The listing builds one solid part. Answer for the finished solid, in the listing's coordinates (mm). Face numbers are marked on the shaded views. A direction names the side the tool comes from. Coordinates: 2 decimals unless noted, no trailing zeros. Write each loop counter-clockwise with the first axis right and the second up, starting at its lowest first coordinate (ties: lowest second). Pieces come first, ordered by that corner, then holes.
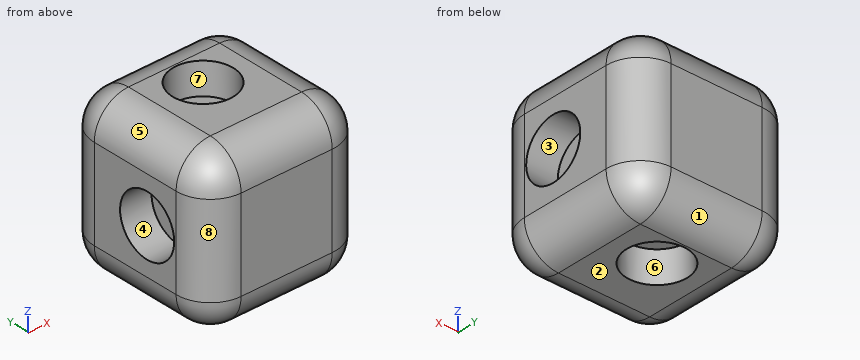
from build123d import *

# Parameters (mm, degrees)
SKETCH1_W                = 29.6037
SKETCH1_H                = 29.6037
BOSS_EXTRUDE1_DEPTH      = 14.80185
BOSS_EXTRUDE1_DEPTH_BACK = 14.80185
FILLET3_R                = 6.35
FILLET4_R                = 6.35
FILLET5_R                = 6.35
FILLET6_R                = 6.35
SKETCH7_R                = 5.588
CUT_EXTRUDE3_DEPTH       = 5.842
SKETCH8_R                = 5.588
CUT_EXTRUDE4_DEPTH       = 5.842
SKETCH3_R                = 5.588
CUT_EXTRUDE5_DEPTH       = 5.842
SKETCH9_R                = 5.588
CUT_EXTRUDE6_DEPTH       = 5.842
FILLET7_R                = 6.35
FILLET8_R                = 6.35


with BuildPart() as part:
    # Sketch1 → Boss-Extrude1 (new body, two sides)
    with BuildSketch(Plane.XY) as boss_extrude1_sk:
        Rectangle(SKETCH1_W, SKETCH1_H)
    extrude(amount=BOSS_EXTRUDE1_DEPTH)
    extrude(boss_extrude1_sk.sketch, amount=-BOSS_EXTRUDE1_DEPTH_BACK)

    # Fillet3
    fillet3_edges = [part.edges().sort_by_distance(p)[0] for p in [
        (14.80185, 14.80185, 0),
    ]]
    fillet(fillet3_edges, radius=FILLET3_R)

    # Fillet4
    fillet4_edges = [part.edges().sort_by_distance(p)[0] for p in [
        (-14.80185, 14.80185, 0),
    ]]
    fillet(fillet4_edges, radius=FILLET4_R)

    # Fillet5
    fillet5_edges = [part.edges().sort_by_distance(p)[0] for p in [
        (-14.80185, -14.80185, 0),
    ]]
    fillet(fillet5_edges, radius=FILLET5_R)

    # Fillet6
    fillet6_edges = [part.edges().sort_by_distance(p)[0] for p in [
        (14.80185, -14.80185, 0),
    ]]
    fillet(fillet6_edges, radius=FILLET6_R)

    # Sketch7 → Cut-Extrude3 (cut)
    with BuildSketch(Plane(origin=(0, 0, -14.80185), x_dir=(-1, 0, 0), z_dir=(0, 0, -1))):
        with Locations((0, 2.47015)):
            Circle(SKETCH7_R)
    extrude(amount=-CUT_EXTRUDE3_DEPTH, mode=Mode.SUBTRACT)

    # Sketch8 → Cut-Extrude4 (cut)
    with BuildSketch(Plane.XY.offset(14.80185)):
        with Locations((0, 2.47015)):
            Circle(SKETCH8_R)
    extrude(amount=-CUT_EXTRUDE4_DEPTH, mode=Mode.SUBTRACT)

    # Sketch3 → Cut-Extrude5 (cut)
    with BuildSketch(Plane.ZY.offset(14.80185)):
        with Locations((0, -2.47015)):
            Circle(SKETCH3_R)
    extrude(amount=-CUT_EXTRUDE5_DEPTH, mode=Mode.SUBTRACT)

    # Sketch9 → Cut-Extrude6 (cut)
    with BuildSketch(Plane(origin=(14.80185, 0, 0), x_dir=(0, 0, -1), z_dir=(1, 0, 0))):
        with Locations((0, -2.47015)):
            Circle(SKETCH9_R)
    extrude(amount=-CUT_EXTRUDE6_DEPTH, mode=Mode.SUBTRACT)

    # Fillet7
    fillet7_edges = [part.edges().sort_by_distance(p)[0] for p in [
        (0, 14.80185, 14.80185),
        (-14.80185, 0, 14.80185),
        (0, -14.80185, 14.80185),
        (14.80185, 0, 14.80185),
    ]]
    fillet(fillet7_edges, radius=FILLET7_R)

    # Fillet8
    fillet8_edges = [part.edges().sort_by_distance(p)[0] for p in [
        (0, 14.80185, -14.80185),
        (-14.80185, 0, -14.80185),
        (0, -14.80185, -14.80185),
        (14.80185, 0, -14.80185),
    ]]
    fillet(fillet8_edges, radius=FILLET8_R)


solid = part.part
Q1. Which of the six approach directions +Z, -Z, +X, -X, +Y, -Y give full straight-line access (tool end or side, diameter ignored) to the marked faces 4, 5, 6, 7 and 8?
Answers below:
face 4: -X
face 5: +Z, -X, +Y, -Y
face 6: -Z
face 7: +Z
face 8: +Z, -Z, -X, -Y
Q2. The part is cut by section D-D, the plane z = 8. Write down the section's boundary in (x, y), then the cut area to 3 significant figures.
Answers below:
outline: (-14.8, -8.45) arc R6.35 ccw to (-8.45, -14.8) - (8.45, -14.8) arc R6.35 ccw to (14.8, -8.45) - (14.8, 8.45) arc R6.35 ccw to (8.45, 14.8) - (-8.45, 14.8) arc R6.35 ccw to (-14.8, 8.45) - close
area: 842 mm2
Q3. Given pin 1 (10 mm diameter, centred on x = 0, y = 2.47, fed in from -Z); pin 2 (1.5 mm diameter, centred on x = 0.5, y = -9.5, fed in from -Z); pin 3 (3 mm diameter, centred on x = -11.5, z = -2, fed in from +Y), each flat-ended and moving along its own axis, determine where each tip first touches the part or whether it passes through.
Answers below:
pin 1: stops at z = -8.96
pin 2: stops at z = -14.79
pin 3: stops at y = 14.61
Q4. The part is cut by section B-B, the plane x = 0. Write down the section's boundary in (y, z).
Answers below:
outline: (-14.8, -8.45) arc R6.35 ccw to (-8.45, -14.8) - (-3.12, -14.8) - (-3.12, -8.96) - (8.06, -8.96) - (8.06, -14.8) - (8.45, -14.8) arc R6.35 ccw to (14.8, -8.45) - (14.8, 8.45) arc R6.35 ccw to (8.45, 14.8) - (8.06, 14.8) - (8.06, 8.96) - (-3.12, 8.96) - (-3.12, 14.8) - (-8.45, 14.8) arc R6.35 ccw to (-14.8, 8.45) - close
Q5. Find the intervals of material crossed by probe 1 along Y at (x, z) = (0, 11.75); probe 2 along Y at (x, z) = (-1.5, -9); probe 3 along X at (y, z) = (1.5, -12), in increasing order.
Answers below:
probe 1: y = -13.88 to -3.12, 8.06 to 13.88
probe 2: y = -14.78 to -2.91, 7.85 to 14.78
probe 3: x = -13.72 to -5.5, 5.5 to 13.72
Q6. Determine the mould class of the marked faces 1, 2 and 3 for opening direction Y: released by +Y, released by -Y, zero draft, split by the parting line, or undercut.
Answers below:
face 1: released by +Y
face 2: zero draft
face 3: undercut
Q7. The part is cut by section A-A, the plane z = 0. Write down the section's boundary in (x, y), then the cut area to 3 significant figures.
Answers below:
outline: (-14.8, -8.45) arc R6.35 ccw to (-8.45, -14.8) - (8.45, -14.8) arc R6.35 ccw to (14.8, -8.45) - (14.8, -8.06) - (8.96, -8.06) - (8.96, 3.12) - (14.8, 3.12) - (14.8, 8.45) arc R6.35 ccw to (8.45, 14.8) - (-8.45, 14.8) arc R6.35 ccw to (-14.8, 8.45) - (-14.8, 3.12) - (-8.96, 3.12) - (-8.96, -8.06) - (-14.8, -8.06) - close
area: 711 mm2
Q8. The part is cut by section C-C, the plane y = 0. Write down the section's boundary in (x, z), then the cut area to 3 significant figures.
Answers below:
outline: (-14.8, -8.45) arc R6.35 ccw to (-8.45, -14.8) - (-5.01, -14.8) - (-5.01, -8.96) - (5.01, -8.96) - (5.01, -14.8) - (8.45, -14.8) arc R6.35 ccw to (14.8, -8.45) - (14.8, -5.01) - (8.96, -5.01) - (8.96, 5.01) - (14.8, 5.01) - (14.8, 8.45) arc R6.35 ccw to (8.45, 14.8) - (5.01, 14.8) - (5.01, 8.96) - (-5.01, 8.96) - (-5.01, 14.8) - (-8.45, 14.8) arc R6.35 ccw to (-14.8, 8.45) - (-14.8, 5.01) - (-8.96, 5.01) - (-8.96, -5.01) - (-14.8, -5.01) - close
area: 608 mm2
